Build history of the part. All positions in model axes, mm. Face numbers are marked on the shaded views. Coordinates: 2 decimals unless noted, no trailing zeros. Order: outer loops, then holes, each group sorted by start corner. A loop starts at its lowest first (then second) coordinate and runs counter-clockwise, first axis right, second up. Notation, with made-up numbers: (-7.75, 36.25) - (45.25, 36.25) arc R27 cw to (45.25, 65.25) - close; hole circle Ø4 at (53, 9.5). An arc over 180 degrees is marked (long way). One line per item, written item: value.
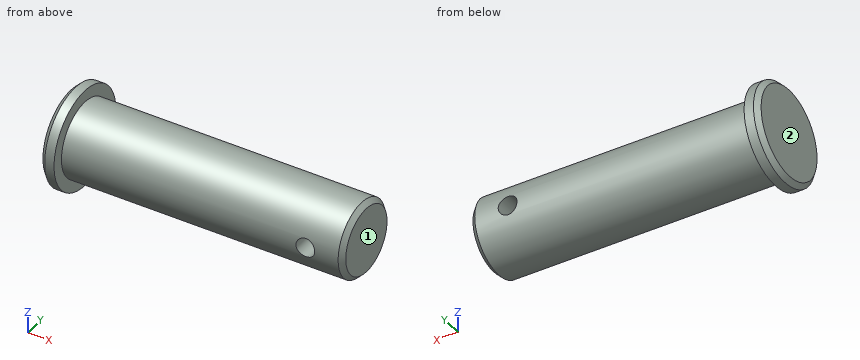
from build123d import *

# Parameters (mm, degrees)
SFAZOWANIE2_SIZE                = 1
SZKIC2_R                        = 2
WYTNIJ_WYCI_GNI_CIE1_DEPTH      = 11.5
WYTNIJ_WYCI_GNI_CIE1_DEPTH_BACK = 11.5


with BuildPart() as part:
    # Szkic1 → Obrót1 (revolve)
    with BuildSketch(Plane.XY):
        Polygon((0, 0), (0, 10.5), (3, 10.5), (3, 8), (63, 8), (63, 0), align=None)
    revolve(axis=Axis((0, 0, 0), (1, 0, 0)))

    # Sfazowanie2
    sfazowanie2_edges = [part.edges().sort_by_distance(p)[0] for p in [
        (0, -10.5, 0),
        (63, -8, 0),
    ]]
    chamfer(sfazowanie2_edges, length=SFAZOWANIE2_SIZE)

    # Szkic2 → Wytnij-wyciągnięcie1 (cut, two sides)
    with BuildSketch(Plane(origin=(0, 0, 0), x_dir=(1, 0, 0), z_dir=(0, 1, 0))) as wytnij_wyci_gni_cie1_sk:
        with Locations((55, 0)):
            Circle(SZKIC2_R)
    extrude(amount=WYTNIJ_WYCI_GNI_CIE1_DEPTH, mode=Mode.SUBTRACT)
    extrude(wytnij_wyci_gni_cie1_sk.sketch, amount=-WYTNIJ_WYCI_GNI_CIE1_DEPTH_BACK, mode=Mode.SUBTRACT)


solid = part.part
1. Two-plate mould, pull along X, no slides. Class the marked faces 1 and 2: pulls with the +X half, pulls with the -X half, needs draft (parallel to the pull), parting line crosses it, or undercut.
Values found:
face 1: pulls with the +X half
face 2: pulls with the -X half
2. Band-saw the part on A-A, the plane z = 0. Give the cut face in (x, y).
Values found:
outline: (0, -9.5) - (1, -10.5) - (3, -10.5) - (3, -8) - (53, -8) - (53, 8) - (3, 8) - (3, 10.5) - (1, 10.5) - (0, 9.5) - close; (57, -8) - (62, -8) - (63, -7) - (63, 7) - (62, 8) - (57, 8) - close
3. Band-saw the part on C-C, the plane x = 15. Give the cut face in (y, z), and give its area (3 significant figures).
Values found:
outline: circle Ø16 at (0, 0)
area: 201 mm2
4. Flat gauge pins, fed straight in: P1, Ø8, axis at x = 49.5, z = 2, coming from the +Y side; P2, Ø1, axis at x = 38.5, y = -1.5, coming from the +Z side; P3, Ø3.5, axis at x = 55, z = 0, coming from the -Y side; P4, Ø4, axis at x = 50.5, y = -5.5, coming from the -Z side. Where does each tip first touch, or does it go through?
Values found:
P1: stops at y = 8
P2: stops at z = 7.94
P3: passes through
P4: stops at z = -7.19
5. Band-saw the part on B-B, the plane x = 55. Give the cut face in (y, z), and give its area (3 significant figures).
Values found:
outline: (-7.75, -2) arc R8 ccw to (7.75, -2) - close; (-7.75, 2) - (7.75, 2) arc R8 ccw to start
area: 138 mm2
6. Probe line 1 along X through (y, z) = (5.75, 0); line 2 along X through (y, z) = (-6, 1.5); line 3 along Z through (x, y) = (55, 3). List the from-to ranges inside material, lowest first.
Values found:
line 1: x = 0 to 53, 57 to 63
line 2: x = 0 to 53.68, 56.32 to 63
line 3: z = -7.42 to -2, 2 to 7.42
